Geometry: final body of the model. Coordinates: model frame, mm. Give positions to 0.01 mm unless a question says otherwise; leave off trailing zeros. Write each loop counter-clockwise with the first axis right and the second up, starting at its lowest first coordinate (ties: lowest second). Pieces come first, ordered by that corner, then holes. Notation, with made-up numbers: M -7.75,65.5 L 8.25,65.5 A25 cw 8.25,83.5 Z; hole C -16,67 d8. An arc over 180 degrees is marked long. One line per question, with ' | ' between items.
from build123d import *

# Parameters (mm, degrees)
EXTRUDE_1_DEPTH     = 10
CUT_EXTRUDE_1_REACH = 50.218
SKETCH_3_R          = 2


with BuildPart() as part:
    # 草图1 → 凸台-拉伸1 (new body)
    with BuildSketch(Plane.XY):
        with BuildLine():
            Line((-3, 0), (-37, 0))
            ThreePointArc((-37, 0), (-39.121320344, 0.878679656), (-40, 3))
            Line((-40, 3), (-40, 22))
            ThreePointArc((-40, 22), (-39.121320344, 24.121320344), (-37, 25))
            Line((-37, 25), (-3, 25))
            ThreePointArc((-3, 25), (-0.878679656, 24.121320344), (0, 22))
            Line((0, 22), (0, 3))
            ThreePointArc((0, 3), (-0.878679656, 0.878679656), (-3, 0))
        make_face()
    extrude(amount=EXTRUDE_1_DEPTH)

    # 草图3 → 切除-拉伸1 (cut, up to next)
    with BuildSketch(Plane.XY.offset(10), mode=Mode.PRIVATE) as cut_extrude_1_sk1:
        with Locations((-30, 19.5)):
            Circle(SKETCH_3_R)
    cut_extrude_1_tool1 = extrude(cut_extrude_1_sk1.sketch, amount=-CUT_EXTRUDE_1_REACH, mode=Mode.PRIVATE) & part.part
    # 草图3 → 切除-拉伸1 (cut, up to next)
    with BuildSketch(Plane.XY.offset(10), mode=Mode.PRIVATE) as cut_extrude_1_sk2:
        with Locations(Location((-30, 5.5, 0), (0, 0, 180))):
            Circle(SKETCH_3_R)
    cut_extrude_1_tool2 = extrude(cut_extrude_1_sk2.sketch, amount=-CUT_EXTRUDE_1_REACH, mode=Mode.PRIVATE) & part.part
    # 草图3 → 切除-拉伸1 (cut, up to next)
    with BuildSketch(Plane.XY.offset(10), mode=Mode.PRIVATE) as cut_extrude_1_sk3:
        with Locations(Location((-10, 19.5, 0), (0, 0, 180))):
            Circle(SKETCH_3_R)
    cut_extrude_1_tool3 = extrude(cut_extrude_1_sk3.sketch, amount=-CUT_EXTRUDE_1_REACH, mode=Mode.PRIVATE) & part.part
    # 草图3 → 切除-拉伸1 (cut, up to next)
    with BuildSketch(Plane.XY.offset(10), mode=Mode.PRIVATE) as cut_extrude_1_sk4:
        with Locations((-10, 5.5)):
            Circle(SKETCH_3_R)
    cut_extrude_1_tool4 = extrude(cut_extrude_1_sk4.sketch, amount=-CUT_EXTRUDE_1_REACH, mode=Mode.PRIVATE) & part.part
    add(cut_extrude_1_tool1.solids().sort_by_distance((-30, 19.5, 10))[0], mode=Mode.SUBTRACT)
    add(cut_extrude_1_tool2.solids().sort_by_distance((-30, 5.5, 10))[0], mode=Mode.SUBTRACT)
    add(cut_extrude_1_tool3.solids().sort_by_distance((-10, 19.5, 10))[0], mode=Mode.SUBTRACT)
    add(cut_extrude_1_tool4.solids().sort_by_distance((-10, 5.5, 10))[0], mode=Mode.SUBTRACT)


solid = part.part
(1) First-contact query: P1, Ø2.5, axis at x = -10, y = 19.5, coming from the -Z side. Flat tip, straight axial feed; report the tip coordinate or a pass-through.
Working result:
P1: passes through
(2) Cut plane B-B, the plane y = 19.5. Return loops of the section in (x, z), then the cut area to 3 significant figures.
Working result:
outline: M -40,0 L -32,0 L -32,10 L -40,10 Z; M -28,0 L -12,0 L -12,10 L -28,10 Z; M -8,0 L 0,0 L 0,10 L -8,10 Z | area: 320 mm^2
(3) Cut plane A-A, the plane x = -30. Return loops of the section in (y, z), then the cut area to 3 significant figures.
Working result:
outline: M 0,0 L 3.5,0 L 3.5,10 L 0,10 Z; M 7.5,0 L 17.5,0 L 17.5,10 L 7.5,10 Z; M 21.5,0 L 25,0 L 25,10 L 21.5,10 Z | area: 170 mm^2
(4) Material intervals for L1, parallel to Y at x = -30, z = 4.75; L2, parallel to X at y = 18.5, z = 9; L3, parallel to Y at x = -11, z = 4.5, sorted ascending. Write a range as [from, to].
Working result:
L1: y = [0, 3.5], [7.5, 17.5], [21.5, 25] | L2: x = [-40, -31.73], [-28.27, -11.73], [-8.27, 0] | L3: y = [0, 3.77], [7.23, 17.77], [21.23, 25]
(5) Cut plane C-C, the plane z = 3.5. Return loops of the section in (x, y).
Working result:
outline: M -40,3 A3 ccw -37,0 L -3,0 A3 ccw 0,3 L 0,22 A3 ccw -3,25 L -37,25 A3 ccw -40,22 Z; hole C -30,5.5 d4; hole C -30,19.5 d4; hole C -10,5.5 d4; hole C -10,19.5 d4
(6) Draft query along Y for faces 1 (the face through (0, 13, 5)), 2 (the face through (-11.474, 6.852, 5.07)), 3 (the face through (-0.9, 24.14, 4.93)). Return one class per face: released by +Y, released by -Y, zero draft, split by the parting line, or undercut.
Working result:
face 1: zero draft | face 2: undercut | face 3: released by +Y
